```python
from build123d import *

# Parameters (mm, degrees)
F0_R      = 17
F1_DEPTH  = 25.4
F2_R      = 21.25
F3_DEPTH  = 25.4
F4_R      = 8.2
F5_DEPTH  = 87.884
F6_W      = 27.94
F6_H      = 6.731
F7_DEPTH  = 25.4
F8_R      = 2.6
F9_DEPTH  = 16.002
F10_W     = 25.4
F10_H     = 6.35
F11_DEPTH = 13.716
F12_R     = 5.08


with BuildPart() as f1:
    # F0 (on Top) → F1 (new body)
    with BuildSketch(Plane.XY):
        Circle(F0_R)
    extrude(amount=F1_DEPTH)

    # F2 (on Top) → F3 (join)
    with BuildSketch(Plane.XY):
        Circle(F2_R)
    extrude(amount=-F3_DEPTH)

    # F4 (on face) → F5 (cut)
    with BuildSketch(Plane(origin=(0, 0, -25.4), x_dir=(1, 0, 0), z_dir=(0, 0, -1))):
        Circle(F4_R)
    extrude(amount=-F5_DEPTH, mode=Mode.SUBTRACT)

    # F6 (on Right) → F7 (cut)
    with BuildSketch(Plane.YZ):
        with Locations((0, -15.182626)):
            Rectangle(F6_W, F6_H)
    extrude(amount=-F7_DEPTH, mode=Mode.SUBTRACT)

    # F8 (on Right) → F9 (cut)
    with BuildSketch(Plane.YZ):
        with Locations((0, -14.992126)):
            Circle(F8_R)
    extrude(amount=F9_DEPTH, mode=Mode.SUBTRACT)

    # F10 (on Right) → F11 (cut)
    with BuildSketch(Plane.YZ):
        with Locations((0, -15.373126)):
            Rectangle(F10_W, F10_H)
    extrude(amount=F11_DEPTH, mode=Mode.SUBTRACT)

    # F12
    f12_edges = [f1.edges().sort_by_distance(p)[0] for p in [
        (-21.25, 0, -25.4),
    ]]
    fillet(f12_edges, radius=F12_R)


solid = f1.part
```
The model under review builds one solid part; all positions refer to its coordinate system, in mm. A direction names the side the tool comes from. Coordinates: 2 decimals unless noted, no trailing zeros. Write each loop counter-clockwise with the first axis right and the second up, starting at its lowest first coordinate (ties: lowest second). Pieces come first, ordered by that corner, then holes. Notation, with made-up numbers: (-8, -1) -> (19, -1) arc R22 cw to (19, 37) -> close; hole circle Ø7 at (44.25, 64). An arc over 180 degrees is marked (long way). One line per item, written item: value. Start each with the question number.
Q1. Add section B-B, the plane z = -8. Give the boundary of the cut face in (x, y).
Q2. To check wall thickness, follow probe 1 along Z at (x, y) = (14.4, 0); probe 2 along Z at (x, y) = (8, -6); probe 3 along Y at (x, z) = (0, 16.5). State the ranges of each line that lie inside material, in increasing order.
Q3. The part is to be moulded in two halves that separate along Y. For faces 4 (the face through (-8, -13.97, -15)), 5 (the face through (7.32, 4.02, 25.4)), 6 (the face through (7, 12.7, -15)), 7 (the face through (20.27, 6.38, -10.02)), say which applies: +Y half, -Y half, draft (parallel to the pull), parting line (faces both ways), or undercut.
Q4. Add section C-C, the plane z = -16.5. Give the boundary of the cut face in (x, y), then the cut area to 3 significant figures.
Q5. Add section A-A, the plane y = 0. Give the boundary of the cut face in (x, z).
Q6. For faces 1 (the face through (-10, 14, 0)), 2 (the face through (10, 0, -12.198)), 3 (the face through (-1.07, -8.13, -22.02)), list the 3-axis set-ups (+Z, -Z, +X, -X, +Y, -Y) from which the entire face can be reached by the end or side of a thin tool; tool diameter is ignored.
Q7. Clearance check with flat-ended pins moving along their axes: P1, Ø3, axis at y = -10.5, z = -15.5, coming from the -X side; P2, Ø5, axis at x = 10.5, z = 10, coming from the -Y side; P3, Ø5.5, axis at x = -7, z = -15.5, coming from the -Y side. State where each tip first meets the part, or that it passes through.
Q8. Add section D-D, the plane z = 8. Give the boundary of the cut face in (x, y), then the cut area to 3 significant figures.
Response:
1. outline: circle Ø42.5 at (0, 0); hole circle Ø16.4 at (0, 0)
2. probe 1: -25.4 to -17.59, -12.39 to 25.4
2. probe 2: -25.4 to -18.55, -12.2 to 25.4
2. probe 3: -17 to -8.2, 8.2 to 17
3. face 4: undercut
3. face 5: draft
3. face 6: undercut
3. face 7: parting line
4. outline: (-16.01, -13.97) arc R21.25 ccw (long way) to (-16.01, 13.97) -> (0, 13.97) -> (0, 12.7) -> (13.72, 12.7) -> (13.72, 2.12) -> (16, 2.12) -> (16, -2.12) -> (13.72, -2.12) -> (13.72, -12.7) -> (0, -12.7) -> (0, -13.97) -> close
4. area: 513 mm²
5. outline: (-21.25, -20.32) arc R5.08 ccw to (-16.17, -25.4) -> (-8.2, -25.4) -> (-8.2, -18.55) -> (-21.25, -18.55) -> close; (-21.25, -11.82) -> (-8.2, -11.82) -> (-8.2, 25.4) -> (-17, 25.4) -> (-17, 0) -> (-21.25, 0) -> close; (8.2, -25.4) -> (16.17, -25.4) arc R5.08 ccw to (21.25, -20.32) -> (21.25, 0) -> (17, 0) -> (17, 25.4) -> (8.2, 25.4) -> (8.2, -12.2) -> (13.72, -12.2) -> (13.72, -12.39) -> (16, -12.39) -> (16, -17.59) -> (13.72, -17.59) -> (13.72, -18.55) -> (8.2, -18.55) -> close
6. face 1: +Z
6. face 2: -X
6. face 3: +Z, -Z
7. P1: x = 13.72
7. P2: y = -15
7. P3: y = -20.82
8. outline: circle Ø34 at (0, 0); hole circle Ø16.4 at (0, 0)
8. area: 697 mm²
